Verification items for this drawing (mm, ordinates from the low corner). A direction names the side the tool comes from. Give positions to 0.01 mm unless a question says otherwise; leave off trailing zeros. Loops run counter-clockwise (first coordinate to the right, second up) from the corner with the lowest first, then second, coordinate; pieces in that order, holes last. Notation, with made-up numbers: M 28,27.5 L 71,27.5 A33 ccw 71,59.5 Z; hole C -7,59.25 d6. An arc over 180 degrees is marked long. Use a Markdown table: item, result.
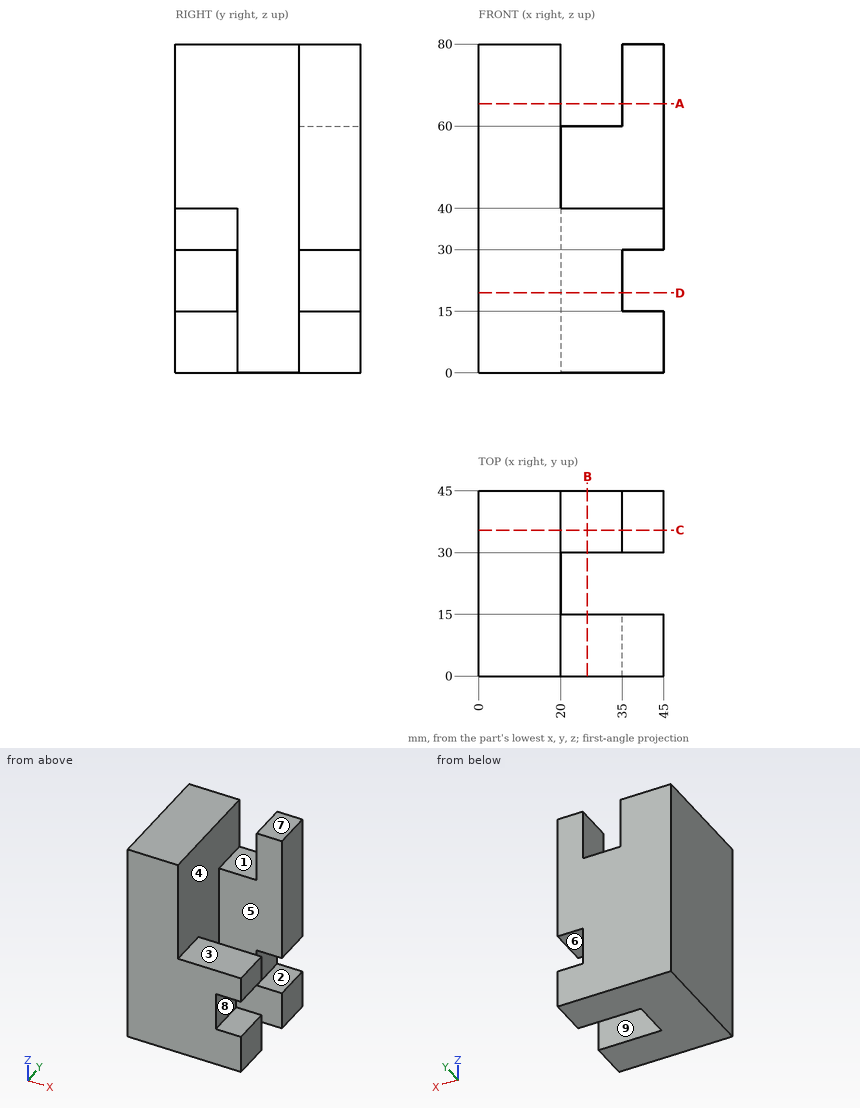
(1) Gauge pin test, flat ends, axial feed: P1, Ø5, axis at x = 42.5, y = 9, coming from the +Z side; P2, Ø7.5, axis at y = 38.5, z = 21, coming from the +X side; P3, Ø7.5, axis at x = 31, y = 38.5, coming from the +Z side. Record the tip position at first contact, or that the pin passes through.
Results below:
| item | result |
|---|---|
| P1 | z = 40 |
| P2 | x = 35 |
| P3 | z = 60 |
(2) Cross-section at D-D on z = 19.5. Record the cut outline in (x, y).
Results below:
| item | result |
|---|---|
| outline | M 0,0 L 35,0 L 35,15 L 20,15 L 20,30 L 35,30 L 35,45 L 0,45 Z |
(3) Draft check along Z on the marked faces 6, 7, 8 and 9. Enter one of: +Z half, -Z half, draft (parallel to the pull), parting line (faces both ways), or undercut.
Results below:
| item | result |
|---|---|
| face 6 | undercut |
| face 7 | +Z half |
| face 8 | undercut |
| face 9 | draft |
(4) Cross-section at B-B on x = 26.5. Record the cut outline in (y, z).
Results below:
| item | result |
|---|---|
| outline | M 0,0 L 15,0 L 15,40 L 0,40 Z; M 30,0 L 45,0 L 45,60 L 30,60 Z |
(5) Material ranges on line 1 (Z direction, x = 40, y = 31); line 2 (Y direction, x = 26.5, z = 46); line 3 (X direction, y = 11, z = 69.5), recorded low to high.
Results below:
| item | result |
|---|---|
| line 1 | 0 to 15, 30 to 80 |
| line 2 | 30 to 45 |
| line 3 | 0 to 20 |
(6) Cross-section at C-C on y = 35.5. Record the cut outline in (x, z), then the cut area to 3 significant figures.
Results below:
| item | result |
|---|---|
| outline | M 0,0 L 45,0 L 45,15 L 35,15 L 35,30 L 45,30 L 45,80 L 35,80 L 35,60 L 20,60 L 20,80 L 0,80 Z |
| area | 3,150 mm^2 |
(7) Set-up check for the marked faces 1, 2, 3, 4 and 5: record each of +Z, -Z, +X, -X, +Y, -Y from which the full face is reachable in a straight line by a thin tool's end or side.
Results below:
| item | result |
|---|---|
| face 1 | +Z, +Y, -Y |
| face 2 | +X, +Y, -Y |
| face 3 | +Z, +X, -Y |
| face 4 | +Z |
| face 5 | +Z, -Z, +X |
(8) Cross-section at A-A on z = 65.5. Record the cut outline in (x, y), then the cut area to 3 significant figures.
Results below:
| item | result |
|---|---|
| outline | M 0,0 L 20,0 L 20,45 L 0,45 Z; M 35,30 L 45,30 L 45,45 L 35,45 Z |
| area | 1,050 mm^2 |
